```python
from build123d import *

# Parameters (mm, degrees)
SKETCH1_W           = 100
SKETCH1_H           = 100
BOSS_EXTRUDE1_DEPTH = 10
BOSS_EXTRUDE2_DEPTH = 10
CUT_EXTRUDE1_DEPTH  = 83.259731469
CIRPATTERN6_COUNT   = 3


with BuildPart() as part:
    # Sketch1 → Boss-Extrude1 (new body)
    with BuildSketch(Plane.XY):
        Rectangle(SKETCH1_W, SKETCH1_H)
    extrude(amount=BOSS_EXTRUDE1_DEPTH)

    # Sketch2 → Boss-Extrude2 (add)
    with BuildSketch(Plane.XY.offset(10)):
        Polygon((-47.749545474, 16.021207549), (-13.108529323, -3.978792451), (-3.108529323, 13.341715625), (-37.749545474, 33.341715625), align=None)
    boss_extrude2 = extrude(amount=BOSS_EXTRUDE2_DEPTH)

    # Sketch3 → Cut-Extrude1 (cut, through all)
    with BuildSketch(Plane(origin=(-8.108529323, 4.681461587, 0), x_dir=(0, 0, -1), z_dir=(0.8660254037844387, -0.4999999999999998, 0))):
        Polygon((-17.5, 5), (-10, 5), (-10, -5), (-17.5, -5), (-17.5, -2.5), (-20, -2.5), (-20, 2.5), (-17.5, 2.5), align=None)
    cut_extrude1 = extrude(amount=-CUT_EXTRUDE1_DEPTH, mode=Mode.SUBTRACT)

    # CirPattern6: Boss-Extrude2, Cut-Extrude1 ×3 about axis
    cirpattern6_axis = Axis((0, 0, 0), (0, 0, 1))
    add([boss_extrude2.rotate(cirpattern6_axis, i * 360 / CIRPATTERN6_COUNT) for i in range(1, CIRPATTERN6_COUNT)])
    add([cut_extrude1.rotate(cirpattern6_axis, i * 360 / CIRPATTERN6_COUNT) for i in range(1, CIRPATTERN6_COUNT)], mode=Mode.SUBTRACT)


solid = part.part
```
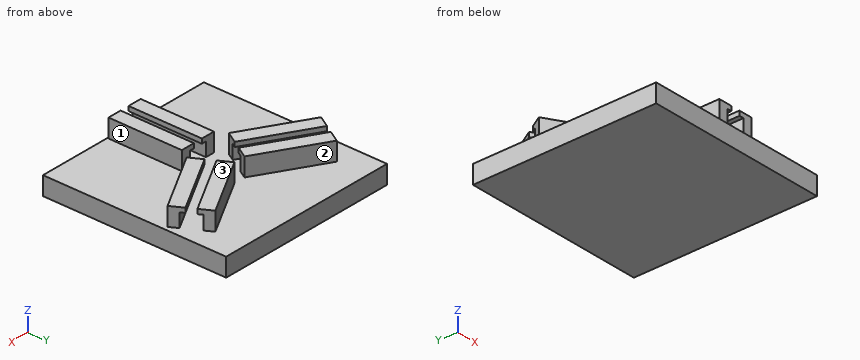
The listing builds one solid part. Answer for the finished solid, in the listing's coordinates (mm). Face numbers are marked on the shaded views. A direction names the side the tool comes from. Coordinates: 2 decimals unless noted, no trailing zeros. Write each loop counter-clockwise with the first axis right and the second up, starting at its lowest first coordinate (ties: lowest second). Pieces come first, ordered by that corner, then holes. Notation, with made-up numbers: (-2, -33) - (6, -33) arc R13 cw to (6, -8) - close; hole circle Ø8 at (-9, -25.5). An arc over 180 degrees is marked (long way). Return JSON: item names as keys, results as strings. Group by question number.
Q1. The part is cut by section C-C on x = -20.5. Write down the section's boundary in (y, z), and give its area (3 significant figures).
Q2. The part is cut by section D-D on y = 35.5. Write down the section's boundary in (x, z).
Q3. The part is cut by section B-B on y = -21. Write down the section's boundary in (x, z).
Q4. Which of the six approach directions +Z, -Z, +X, -X, +Y, -Y give full straight-line access (tool end or side, diameter ignored) to the marked faces 1, 2 and 3?
Q5. The part is cut by section A-A on z = 16. Write down the section's boundary in (x, y).
Q6. Find the intervals of material crossed by line 1 along X through (y, z) = (-28.5, 12.5); line 2 along X through (y, z) = (7, 19.25); line 3 along Z through (x, y) = (4, -11), in increasing order. Write a range as [from, to].
Q7. Flat-ended cylindrical pins translate along their axes: pin 1 Ø2 at (y, z) = (-30, 19) entering from +X; pin 2 Ø11 at (y, z) = (-30.5, 17) entering from -X; pin 3 Ø5 at (x, y) = (31, 1) entering from +Z. Find the tip coordinate at first contact, or state that the pin passes through.
Evaluation:
{
 "1": {"outline": "(-50, 0) - (50, 0) - (50, 10) - (23.38, 10) - (23.38, 20) - (14.72, 20) - (14.72, 17.5) - (17.61, 17.5) - (17.61, 10) - (6.06, 10) - (6.06, 17.5) - (8.95, 17.5) - (8.95, 20) - (0.29, 20) - (0.29, 10) - (-50, 10) - close", "area": "1,130 mm2"},
 "2": {"outline": "(-50, 0) - (50, 0) - (50, 10) - (-50, 10) - close"},
 "3": {"outline": "(-50, 0) - (50, 0) - (50, 10) - (10, 10) - (10, 20) - (2.5, 20) - (2.5, 17.5) - (5, 17.5) - (5, 10) - (-5, 10) - (-5, 17.5) - (-2.5, 17.5) - (-2.5, 20) - (-10, 20) - (-10, 10) - (-50, 10) - close"},
 "4": {"face 1": "+Z, +X, -Y", "face 2": "+Z, +Y", "face 3": "+Z, +X, -X, +Y, -Y"},
 "5": {"outline": "(-47.75, 16.02) - (-13.11, -3.98) - (-10.61, 0.35) - (-45.25, 20.35) - close; (-40.25, 29.01) - (-5.61, 9.01) - (-3.11, 13.34) - (-37.75, 33.34) - close; (-10, -49.36) - (-5, -49.36) - (-5, -9.36) - (-10, -9.36) - close; (3.11, 13.34) - (5.61, 9.01) - (40.25, 29.01) - (37.75, 33.34) - close; (5, -49.36) - (10, -49.36) - (10, -9.36) - (5, -9.36) - close; (10.61, 0.35) - (13.11, -3.98) - (47.75, 16.02) - (45.25, 20.35) - close"},
 "6": {"line 1": "x = [-10, -5], [5, 10]", "line 2": "x = [-32.12, -17.12], [-7.12, -6.77], [6.77, 7.12], [17.12, 32.12]", "line 3": "z = [0, 10], [17.5, 20]"},
 "7": {"pin 1": "stops at x = 10", "pin 2": "stops at x = -10", "pin 3": "stops at z = 10"}
}
